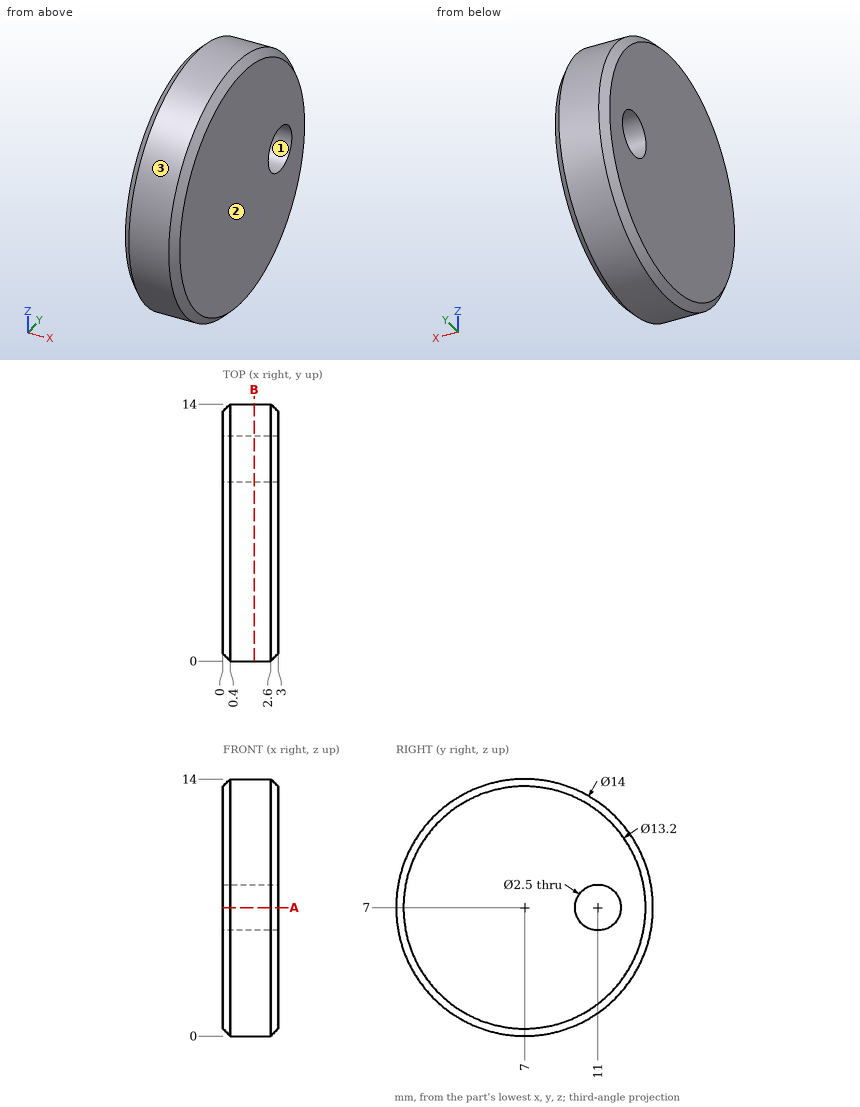
Geometry check sheet. Reference: drawing and pictorial views, mm from the part's lowest x, y, z. Give positions to 0.01 mm unless a question says otherwise; leave off trailing zeros. Order: outer loops, then holes, each group sorted by start corner. A loop starts at its lowest first (then second) coordinate and runs counter-clockwise, first axis right, second up. Notation, with made-up numbers: M 60,12 L 113,12 A28 cw 113,38 Z; hole C -39,61 d1. An arc over 180 degrees is marked long. Answer as CSV lines item,"result". Start each with the question number.
Item 1: Mould release check, pull along Y, two halves, no side actions. Record for the marked faces 1, 2 and 3: +Y half, -Y half, draft (parallel to the pull), parting line (faces both ways), or undercut.
Item 2: Cross-section at A-A on z = 7. Enter the section's corners in (x, y).
Item 3: Gauge pin test, flat ends, axial feed: P1, Ø3, axis at y = 4, z = 8.5, coming from the -X side; P2, Ø1, axis at x = 0.5, z = 10.5, coming from the +Y side. Record the tip position at first contact, or that the pin passes through.
Item 4: Thickness scan on line 1 (Z direction, x = 1.7, y = 10.25); line 2 (Y direction, x = 0.55, z = 6); line 3 (Z direction, x = 2.85, y = 8). Record the ranges inside material, lowest first. Write a range as [from, to].
Item 5: Cross-section at B-B on x = 1.7. Enter the section's corners in (y, z).
Established:
1,face 1,"undercut"
1,face 2,"draft"
1,face 3,"parting line"
2,outline,"M 0,0.4 L 0.4,0 L 2.6,0 L 3,0.4 L 3,9.75 L 0,9.75 Z; M 0,12.25 L 3,12.25 L 3,13.6 L 2.6,14 L 0.4,14 L 0,13.6 Z"
3,P1,"stops at x = 0"
3,P2,"stops at y = 13.32"
4,line 1,"z = [0.8, 6], [8, 13.2]"
4,line 2,"y = [0.07, 10.25], [11.75, 13.93]"
4,line 3,"z = [0.32, 13.68]"
5,outline,"C 7,7 d14; hole C 11,7 d2.5"
